```python
from build123d import *


with BuildPart() as part:
    # Sketch1 → Revolve1 (revolve)
    with BuildSketch(Plane.YZ, mode=Mode.PRIVATE) as revolve1_sk:
        Polygon((6, 0), (6, 7.5), (1.5, 7.5), (1.5, 27.5), (6, 27.5), (6, 32.5), (-6, 32.5), (-6, 27.5), (-1.5, 27.5), (-1.5, 7.5), (-8, 7.5), (-8, 0), align=None)
    revolve(revolve1_sk.sketch.rotate(Axis((0, 0, 0), (0, 1, 0)), 180), axis=Axis((0, 0, 0), (0, 1, 0)))


solid = part.part
```
Model file for the job. Use its own axes, mm. A direction names the side the tool comes from. Give positions to 0.01 mm unless a question says otherwise; leave off trailing zeros. Order: outer loops, then holes, each group sorted by start corner. A loop starts at its lowest first (then second) coordinate and runs counter-clockwise, first axis right, second up.
1) Saw through at B-B, the plane x = 0. Write the cut outline in (y, z), then the cut area to 3 significant figures.
2) Saw through at C-C, the plane z = 0. Write the cut outline in (x, y), then the cut area to 3 significant figures.
3) Wall check: probe 1 along X at (y, z) = (2.25, 0); probe 2 along Z at (x, y) = (-1, 2.5); probe 3 along Z at (x, y) = (-2, -5.75). Give the ranges that are in metal, low to high.
4) Saw through at D-D, the plane y = -7. Write the cut outline in (x, z), then the cut area to 3 significant figures.
5) Pin check, flat tips, straight feed: pin 1 (10 mm diameter, centred on x = 0.5, z = 24, fed in from +Y); pin 2 (1.5 mm diameter, centred on x = 7, z = 6.5, fed in from -Y); pin 3 (1 mm diameter, centred on y = 1.5, z = 17.5, fed in from -X); pin 4 (1.5 mm diameter, centred on y = 0.5, z = 25.5, fed in from -X). Stop position of each tip, or through.
6) 3-axis set-ups, long thin cutter, end or side, ignore diameter. For faces 1 (the flat face through (0, 6, 0)), 2 (the cylindrical face through (24.397, -3.718, -12.69)), 3 (the cylindrical face through (-6.324, 3.718, -4.032)): which of +Z, -Z, +X, -X, +Y, -Y reach the whole face in a straight line?
7) Mould opens along X. For faces 4 (the cylindrical face through (-9.76, -0.08, -31)), 5 (the flat face through (-7, 6, -27)), 6 (the flat face through (6, 1.5, 6)) say: +X half, -X half, draft (parallel to the pull), parting line (faces both ways), or undercut.
8) Saw through at A-A, the plane y = -2.25. Write the cut outline in (x, z), then the cut area to 3 significant figures.
Computed:
1. outline: (-8, -7.5) - (-1.5, -7.5) - (-1.5, -27.5) - (-6, -27.5) - (-6, -32.5) - (6, -32.5) - (6, -27.5) - (1.5, -27.5) - (1.5, -7.5) - (6, -7.5) - (6, 7.5) - (1.5, 7.5) - (1.5, 27.5) - (6, 27.5) - (6, 32.5) - (-6, 32.5) - (-6, 27.5) - (-1.5, 27.5) - (-1.5, 7.5) - (-8, 7.5) - close
1. area: 450 mm2
2. outline: (-32.5, -6) - (-27.5, -6) - (-27.5, -1.5) - (-7.5, -1.5) - (-7.5, -8) - (7.5, -8) - (7.5, -1.5) - (27.5, -1.5) - (27.5, -6) - (32.5, -6) - (32.5, 6) - (27.5, 6) - (27.5, 1.5) - (7.5, 1.5) - (7.5, 6) - (-7.5, 6) - (-7.5, 1.5) - (-27.5, 1.5) - (-27.5, 6) - (-32.5, 6) - close
2. area: 450 mm2
3. probe 1: x = -32.5 to -27.5, -7.5 to 7.5, 27.5 to 32.5
3. probe 2: z = -32.48 to -27.48, -7.43 to 7.43, 27.48 to 32.48
3. probe 3: z = -32.44 to -27.43, -7.23 to 7.23, 27.43 to 32.44
4. outline: circle Ø15 at (0, 0)
4. area: 177 mm2
5. pin 1: stops at y = 6
5. pin 2: stops at y = -1.5
5. pin 3: stops at x = -27.7
5. pin 4: stops at x = -21.06
6. face 1: +Z, -Z, +X, -X, +Y
6. face 2: -Y
6. face 3: +Y
7. face 4: parting line
7. face 5: draft
7. face 6: undercut
8. outline: circle Ø65 at (0, 0); circle Ø15 at (0, 0); hole circle Ø55 at (0, 0)
8. area: 1,120 mm2
